Can you work these out from the drawing? Everything is in mm from the part's minimum corner. Coordinates: 2 decimals unless noted, no trailing zeros. Loops run counter-clockwise (first coordinate to the right, second up) from the corner with the lowest first, then second, coordinate; pieces in that order, holes last. Notation, with made-up numbers: (76.5, 3.25) -> (129.5, 3.25) arc R5 ccw to (129.5, 9.25) -> close; hole circle Ø10 at (-6.5, 70.5). An arc over 180 degrees is marked (long way). Put each result on its own line as item: value. Start each with the question number.
Item 1: If we section it at D-D on y = 0.9: Please give me the cut outline in (x, z) (1 decimal), plus the area to 3 significant figures.
Item 2: Please list where these lines run through material, in increasing order: L1, parallel to X at y = 1.8, z = 34; L2, parallel to X at y = 2.8, z = 31 (1 decimal); L3, parallel to X at y = 3.1, z = 24 (1 decimal). Write a range as from..to.
Item 3: If we section it at A-A on z = 34: Please give me the cut outline in (x, y).
Item 4: Will this pin go through, and if not, where does the flat tip stop? P1, Ø1.5, axis at x = 32.5, y = 2, coming from the -Z side (1 decimal).
Item 5: If we section it at B-B on x = 23.5: Please give me the cut outline in (y, z) (1 decimal), plus the area to 3 significant figures.
Item 6: We'd pull the mould along Z, two halves only. Please class the marked faces 1, 2 and 3: pulls with the +Z half, pulls with the -Z half, needs draft (parallel to the pull), parting line crosses it, or undercut.
Item 7: If we section it at C-C on z = 26.5: Please give me the cut outline in (x, y).
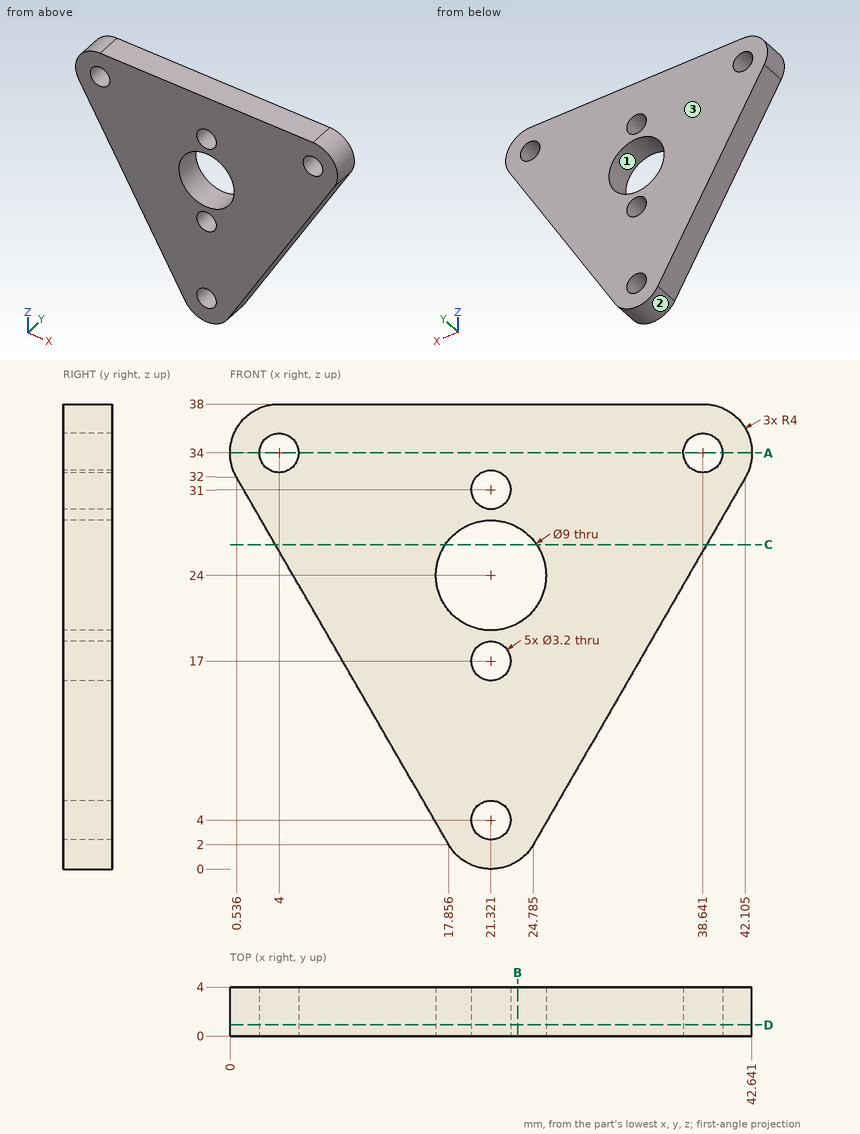
Solutions:
1. outline: (0.5, 32) -> (17.9, 2) arc R4 ccw to (24.8, 2) -> (42.1, 32) arc R4 ccw to (38.6, 38) -> (4, 38) arc R4 ccw to start; hole circle Ø3.2 at (4, 34); hole circle Ø9 at (21.3, 24); hole circle Ø3.2 at (21.3, 4); hole circle Ø3.2 at (21.3, 17); hole circle Ø3.2 at (21.3, 31); hole circle Ø3.2 at (38.6, 34)
1. area: 882 mm^2
2. L1: 0..2.4, 5.6..37.04, 40.24..42.64
2. L2: 1.1..19.7, 22.9..41.5
2. L3: 5.2..16.8, 25.8..37.5
3. outline: (0, 0) -> (2.4, 0) -> (2.4, 4) -> (0, 4) -> close; (5.6, 0) -> (37.04, 0) -> (37.04, 4) -> (5.6, 4) -> close; (40.24, 0) -> (42.64, 0) -> (42.64, 4) -> (40.24, 4) -> close
4. P1: z = 14.1
5. outline: (0, 0.6) -> (4, 0.6) -> (4, 20.1) -> (0, 20.1) -> close; (0, 27.9) -> (4, 27.9) -> (4, 38) -> (0, 38) -> close
5. area: 118 mm^2
6. face 1: undercut
6. face 2: pulls with the -Z half
6. face 3: needs draft
7. outline: (3.71, 0) -> (17.58, 0) -> (17.58, 4) -> (3.71, 4) -> close; (25.06, 0) -> (38.93, 0) -> (38.93, 4) -> (25.06, 4) -> close
